Here's how the part is built. I have some questions about the finished solid (model axes, mm). Face numbers are marked on the shaded views. Give positions to 0.01 mm unless a question says otherwise; leave off trailing zeros. Write each loop counter-clockwise with the first axis right and the second up, starting at its lowest first coordinate (ties: lowest second). Pieces come first, ordered by that corner, then holes. Notation, with made-up numbers: M -34,35.5 L -28,35.5 A23 cw -28,47.5 Z; hole C 83.5,81.5 d5. An arc over 180 degrees is marked long. Use one line per item in the form item = value. Start each with the question number.
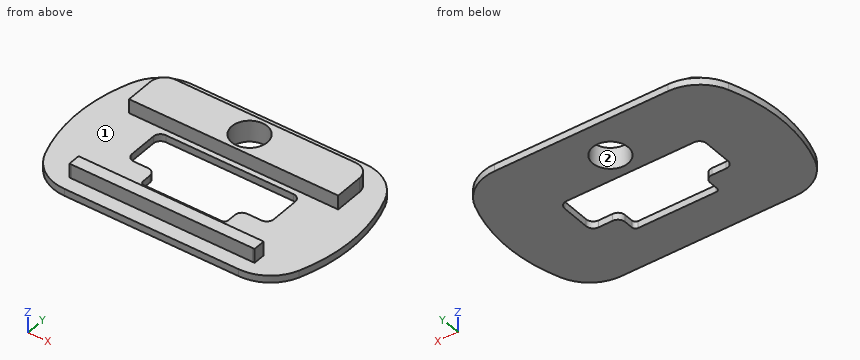
from build123d import *

# Parameters (mm, degrees)
BOSS_EXTRUDE1_DEPTH     = 1
BOSS_EXTRUDE2_DEPTH     = 3
CUT_EXTRUDE3_DEPTH      = 3
SKETCH7_W               = 29.714207492
SKETCH7_H               = 11.789960261
CUT_EXTRUDE4_DEPTH      = 2
CUT_EXTRUDE5_DEPTH      = 33.440982602
CUT_EXTRUDE5_DEPTH_BACK = 33.440982602
SKETCH6_R               = 2.5


with BuildPart() as part:
    # Sketch4 → Boss-Extrude1 (new body)
    with BuildSketch(Plane.XY):
        with BuildLine():
            Line((-11.46999612, 1.189613235), (13.12949411, 1.189613235))
            ThreePointArc((13.12949411, 1.189613235), (16.545477006, 2.256960718), (18.746112986, 5.079259617))
            add(Edge.make_bspline(
                [(18.746112986, 5.079259617), (19.737187318, 7.716962964), (20.720796973, 13.218046534), (19.706022352, 18.616089167), (18.698180615, 21.299335004)],
                knots=[0.167422492, 0.167422492, 0.167422492, 0.167422492, 0.502499344, 0.837905074, 0.837905074, 0.837905074, 0.837905074], degree=3))
            ThreePointArc((18.698180615, 21.299335004), (16.497584709, 24.122073606), (13.081324372, 25.189613235))
            Line((13.081324372, 25.189613235), (-11.421826382, 25.189613235))
            ThreePointArc((-11.421826382, 25.189613235), (-14.838086719, 24.122073606), (-17.038682625, 21.299335004))
            add(Edge.make_bspline(
                [(-17.086614996, 5.079259617), (-18.077689328, 7.716962964), (-19.061298983, 13.218046534), (-18.046524362, 18.616089167), (-17.038682625, 21.299335004)],
                knots=[0.167422492, 0.167422492, 0.167422492, 0.167422492, 0.502499344, 0.837905074, 0.837905074, 0.837905074, 0.837905074], degree=3))
            ThreePointArc((-17.086614996, 5.079259617), (-14.885979016, 2.256960718), (-11.46999612, 1.189613235))
        make_face()
    extrude(amount=BOSS_EXTRUDE1_DEPTH)

    # Sketch1 → Boss-Extrude2 (add)
    with BuildSketch(Plane.XY):
        with BuildLine():
            Line((-11.928396375, 3.192285122), (13.571603625, 3.192285122))
            ThreePointArc((13.571603625, 3.192285122), (13.725432705, 3.198209744), (13.878350405, 3.215948508))
            Line((13.878350405, 3.215948508), (13.878350405, 6.42715263))
            ThreePointArc((13.878350405, 6.42715263), (14.024797015, 6.780706021), (14.378350405, 6.92715263))
            Line((14.378350405, 6.92715263), (15.571603625, 6.92715263))
            Line((15.571603625, 6.92715263), (15.571603625, 20.692285122))
            ThreePointArc((15.571603625, 20.692285122), (14.985817187, 22.106498684), (13.571603625, 22.692285122))
            Line((13.571603625, 22.692285122), (-11.928396375, 22.692285122))
            ThreePointArc((-11.928396375, 22.692285122), (-13.342609938, 22.106498684), (-13.928396375, 20.692285122))
            Line((-13.928396375, 20.692285122), (-13.928396375, 6.92715263))
            Line((-13.928396375, 6.92715263), (-12.735143156, 6.92715263))
            ThreePointArc((-12.735143156, 6.92715263), (-12.381589765, 6.780706021), (-12.235143156, 6.42715263))
            Line((-12.235143156, 6.42715263), (-12.235143156, 3.215948508))
            ThreePointArc((-12.235143156, 3.215948508), (-12.082225455, 3.198209744), (-11.928396375, 3.192285122))
        make_face()
    extrude(amount=BOSS_EXTRUDE2_DEPTH)

    # Sketch2 → Cut-Extrude3 (cut)
    with BuildSketch(Plane.XY):
        with BuildLine():
            Line((-4.678396375, 7.121027254), (6.321603625, 7.121027254))
            ThreePointArc((6.321603625, 7.121027254), (6.675157015, 7.267473863), (6.821603625, 7.621027254))
            Line((6.821603625, 7.621027254), (6.821603625, 8.901007801))
            ThreePointArc((6.821603625, 8.901007801), (7.114496843, 9.608114582), (7.821603625, 9.901007801))
            Line((7.821603625, 9.901007801), (9.821603625, 9.901007801))
            ThreePointArc((9.821603625, 9.901007801), (10.528710406, 10.19390102), (10.821603625, 10.901007801))
            Line((10.821603625, 10.901007801), (10.821603625, 14.92428318))
            ThreePointArc((10.821603625, 14.92428318), (10.528710406, 15.631389961), (9.821603625, 15.92428318))
            Line((9.821603625, 15.92428318), (-8.178396375, 15.92428318))
            ThreePointArc((-8.178396375, 15.92428318), (-8.885503157, 15.631389961), (-9.178396375, 14.92428318))
            Line((-9.178396375, 14.92428318), (-9.178396375, 10.901007801))
            ThreePointArc((-9.178396375, 10.901007801), (-8.885503157, 10.19390102), (-8.178396375, 9.901007801))
            Line((-8.178396375, 9.901007801), (-6.178396375, 9.901007801))
            ThreePointArc((-6.178396375, 9.901007801), (-5.471289594, 9.608114582), (-5.178396375, 8.901007801))
            Line((-5.178396375, 8.901007801), (-5.178396375, 7.621027254))
            ThreePointArc((-5.178396375, 7.621027254), (-5.031949766, 7.267473863), (-4.678396375, 7.121027254))
        make_face()
    extrude(amount=CUT_EXTRUDE3_DEPTH, mode=Mode.SUBTRACT)

    # Sketch7 → Cut-Extrude4 (cut)
    with BuildSketch(Plane.XY.offset(3)):
        with Locations((0.928707371, 10.792421827)):
            Rectangle(SKETCH7_W, SKETCH7_H)
    extrude(amount=-CUT_EXTRUDE4_DEPTH, mode=Mode.SUBTRACT)

    # Sketch6 → Cut-Extrude5 (cut, two sides: drawn at the far end of the back side and taken through both)
    with BuildSketch(Plane.XY.offset(3).offset(-CUT_EXTRUDE5_DEPTH_BACK)):
        with Locations((0.821603625, 19.685063144)):
            Circle(SKETCH6_R)
    extrude(amount=CUT_EXTRUDE5_DEPTH + CUT_EXTRUDE5_DEPTH_BACK, mode=Mode.SUBTRACT)


solid = part.part
1) Will these pins go through, and if not, where does the flat tip stop? P1, Ø1, axis at x = 1.5, z = 2.5, coming from the -Y side; P2, Ø1.1, axis at y = 8, z = 0.5, coming from the -X side; P3, Ø1.3, axis at y = 4, z = 2, coming from the +X side; P4, Ø3, axis at x = 0.82, y = 19.69, coming from the -Z side.
2) Suppose I cut it at C-C, the plane x = 11.5. List the corners of the cut face in (y, z) for me.
3) Suppose I cut it at A-A, the plane z = 2.1. List the corners of the cut face in (x, y) for me.
4) Suppose I cut it at D-D, the plane x = -15. List the corners of the cut face in (y, z) for me, and give its area (3 significant figures).
5) Suppose I cut it at B-B, the plane x = -3. List the corners of the cut face in (y, z) for me.
6) Please list where these lines run through material, in increasing order: line 1 (Y direction, x = -11, z = 1.5); line 2 (Y direction, x = -0.5, z = 0.6); line 3 (Y direction, x = -7, z = 0.35).
7) Thinking about a two-plate mould opening in X: for the marked faces 1 and 2, which applies, released by +X, released by -X, zero draft, split by the parting line, or undercut?
Checks:
q1.P1 = 3.19
q1.P2 = -18.09
q1.P3 = 13.88
q1.P4 = through
q2.outline = M 1.19,0 L 25.19,0 L 25.19,1 L 22.69,1 L 22.69,3 L 16.69,3 L 16.69,1 L 4.9,1 L 4.9,3 L 3.19,3 L 3.19,1 L 1.19,1 Z
q3.outline = M -13.93,16.69 L 15.57,16.69 L 15.57,20.69 A2 ccw 13.57,22.69 L -11.93,22.69 A2 ccw -13.93,20.69 Z; M -12.24,3.22 A2 ccw -11.93,3.19 L 13.57,3.19 A2 ccw 13.88,3.22 L 13.88,4.9 L -12.24,4.9 Z; hole C 0.82,19.69 d5
q4.outline = M 2.34,0 L 24.01,0 L 24.01,1 L 2.34,1 Z
q4.area = 21.7 mm^2
q5.outline = M 1.19,0 L 7.12,0 L 7.12,1 L 4.9,1 L 4.9,3 L 3.19,3 L 3.19,1 L 1.19,1 Z; M 15.92,0 L 25.19,0 L 25.19,1 L 22.69,1 L 22.69,3 L 16.69,3 L 16.69,1 L 15.92,1 Z
q6.line_1 = 3.19 to 4.9, 16.69 to 22.69
q6.line_2 = 1.19 to 7.12, 15.92 to 17.56, 21.81 to 25.19
q6.line_3 = 1.19 to 9.9, 15.92 to 25.19
q7.face_1 = zero draft
q7.face_2 = undercut
